For this review, take the finished solid that the model builds, in its own axes (mm). Round coordinates to 2 decimals unless told otherwise and drop trailing zeros. Order: outer loops, then holes, each group sorted by start corner. A loop starts at its lowest first (then second) coordinate and runs counter-clockwise, first axis right, second up. Notation, with made-up numbers: M 41.5,70 L 85.5,70 A21 ccw 85.5,88 Z; hole C 55.25,-23.75 d1. An arc over 180 degrees is marked long. Answer as a JSON object with one key per item and string values.
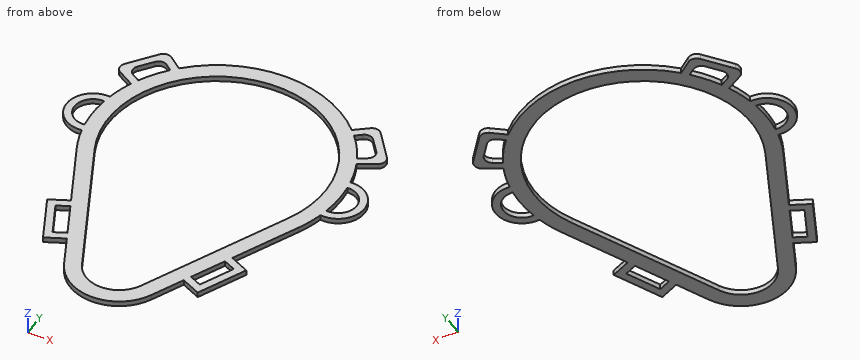
from build123d import *

# Parameters (mm, degrees)
BOSS_EXTRUDE1_DEPTH = 2
BOSS_EXTRUDE2_DEPTH = 2
BOSS_EXTRUDE3_DEPTH = 2
BOSS_EXTRUDE4_DEPTH = 2


with BuildPart() as part:
    # Sketch1 → Boss-Extrude1 (new body)
    with BuildSketch(Plane.XY):
        with BuildLine():
            Line((-42.535849019, -19.992537313), (-16.742834188, -74.869402985))
            ThreePointArc((-16.742834188, -74.869402985), (0, -85.5), (16.742834188, -74.869402985))
            Line((16.742834188, -74.869402985), (42.535849019, -19.992537313))
            ThreePointArc((42.535849019, -19.992537313), (0, 47), (-42.535849019, -19.992537313))
        make_face()
        with BuildLine():
            Line((37.105740634, -17.440298507), (11.312725803, -72.317164179))
            ThreePointArc((11.312725803, -72.317164179), (0, -79.5), (-11.312725803, -72.317164179))
            Line((-11.312725803, -72.317164179), (-37.105740634, -17.440298507))
            ThreePointArc((-37.105740634, -17.440298507), (0, 41), (37.105740634, -17.440298507))
        make_face(mode=Mode.SUBTRACT)
    extrude(amount=BOSS_EXTRUDE1_DEPTH)

    # Sketch2 → Boss-Extrude2 (add)
    # profile 1 of 2: a face of its own
    with BuildSketch(Plane.XY.offset(2)):
        Polygon((38.155605521, -48.118901031), (29.648142834, -66.219262316), (19.692944127, -61.540157838), (28.200406814, -43.439796554), align=None)
        Polygon((29.639341604, -47.430970149), (34.164431925, -49.557835821), (28.209208044, -62.22808872), (23.684117723, -60.101223049), align=None, mode=Mode.SUBTRACT)
    # profile 2 of 2: a face of its own
    with BuildSketch(Plane.XY.offset(2)):
        Polygon((-28.200406814, -43.439796554), (-38.155605521, -48.118901031), (-29.648142834, -66.219262316), (-19.692944127, -61.540157838), align=None)
        Polygon((-29.639341604, -47.430970149), (-23.684117723, -60.101223049), (-28.209208044, -62.22808872), (-34.164431925, -49.557835821), align=None, mode=Mode.SUBTRACT)
    extrude(amount=-BOSS_EXTRUDE2_DEPTH)

    # Sketch3 → Boss-Extrude3 (add)
    # profile 1 of 2: a face of its own
    with BuildSketch(Plane.XY.offset(2)):
        with BuildLine():
            Line((-31.151373165, 31.772817784), (-38.114457897, 37.177116489))
            ThreePointArc((-38.114457897, 37.177116489), (-40.329006137, 37.783626199), (-42.323795344, 36.64657125))
            Line((-42.323795344, 36.64657125), (-50.184128352, 26.519047267))
            ThreePointArc((-50.184128352, 26.519047267), (-50.760622602, 24.115277799), (-49.336666072, 22.094683561))
            Line((-49.336666072, 22.094683561), (-41.03528616, 17.205385487))
            Line((-41.03528616, 17.205385487), (-31.151373165, 31.772817784))
        make_face()
        with BuildLine():
            Line((-35.213971315, 31.128382936), (-37.583912658, 32.967779041))
            ThreePointArc((-37.583912658, 32.967779041), (-39.798460899, 33.574288752), (-41.793250106, 32.437233803))
            Line((-41.793250106, 32.437233803), (-45.72341661, 27.373471811))
            ThreePointArc((-45.72341661, 27.373471811), (-46.29991086, 24.969702343), (-44.87595433, 22.949108105))
            Line((-44.87595433, 22.949108105), (-41.937721652, 21.218565047))
            Line((-41.937721652, 21.218565047), (-35.213971315, 31.128382936))
        make_face(mode=Mode.SUBTRACT)
    # profile 2 of 2: a face of its own
    with BuildSketch(Plane.XY.offset(2)):
        with BuildLine():
            Line((31.151373165, 31.772817784), (41.03528616, 17.205385487))
            Line((41.03528616, 17.205385487), (49.521231884, 22.082259987))
            ThreePointArc((49.521231884, 22.082259987), (50.972840228, 24.118942465), (50.376596508, 26.547879626))
            Line((50.376596508, 26.547879626), (42.329184832, 36.691250185))
            ThreePointArc((42.329184832, 36.691250185), (40.338269585, 37.80509541), (38.139596853, 37.19662773))
            Line((38.139596853, 37.19662773), (31.151373165, 31.772817784))
        make_face()
        with BuildLine():
            Line((35.213971315, 31.128382936), (41.937721652, 21.218565047))
            Line((41.937721652, 21.218565047), (44.9588763, 22.954823155))
            ThreePointArc((44.9588763, 22.954823155), (46.410484644, 24.991505634), (45.814240924, 27.420442794))
            Line((45.814240924, 27.420442794), (41.798639593, 32.481912737))
            ThreePointArc((41.798639593, 32.481912737), (39.807724347, 33.595757962), (37.609051614, 32.987290283))
            Line((37.609051614, 32.987290283), (35.213971315, 31.128382936))
        make_face(mode=Mode.SUBTRACT)
    extrude(amount=-BOSS_EXTRUDE3_DEPTH)

    # Sketch4 → Boss-Extrude4 (add)
    # profile 1 of 2: a face of its own
    with BuildSketch(Plane.XY.offset(2)):
        with BuildLine():
            Line((42.848392472, 8.262286082), (42.848392472, -9.939496711))
            ThreePointArc((42.848392472, -9.939496711), (56.992517927, -0.838605315), (42.848392472, 8.262286082))
        make_face()
        with BuildLine():
            Line((45.848392472, 6.067260087), (45.848392472, -7.744470716))
            ThreePointArc((45.848392472, -7.744470716), (53.992517927, -0.838605315), (45.848392472, 6.067260087))
        make_face(mode=Mode.SUBTRACT)
    # profile 2 of 2: a face of its own
    with BuildSketch(Plane.XY.offset(2)):
        with BuildLine():
            Line((-42.848392472, 8.262286082), (-42.848392472, -9.939496711))
            ThreePointArc((-42.848392472, -9.939496711), (-56.992517927, -0.838605315), (-42.848392472, 8.262286082))
        make_face()
        with BuildLine():
            Line((-45.848392472, 6.067260087), (-45.848392472, -7.744470716))
            ThreePointArc((-45.848392472, -7.744470716), (-53.992517927, -0.838605315), (-45.848392472, 6.067260087))
        make_face(mode=Mode.SUBTRACT)
    extrude(amount=-BOSS_EXTRUDE4_DEPTH)


solid = part.part
1) Add section B-B on y = 0. State the section outline as (x, z) points, and give its area (3 significant figures).
Geometry check:
{"outline": "M -56.96,0 L -53.94,0 L -53.94,2 L -56.96,2 Z; M -47,0 L -41,0 L -41,2 L -47,2 Z; M 41,0 L 47,0 L 47,2 L 41,2 Z; M 53.94,0 L 56.96,0 L 56.96,2 L 53.94,2 Z", "area": "36.1 mm²"}
2) Add section D-D on z = 0.5. State how many separate pieces and enclosed holes the cut face has, and give its area (3 significant figures).
Geometry check:
{"separate pieces": "1", "enclosed holes": "7", "area": "2,540 mm²"}
3) For L1, parallel to X at y = 0, z = 1; L2, parallel to Y at x = -31.5, z = 1.25; L3, parallel to X at y = -48.5, z = 1.4, list the stretches that pass through material, from the lowest coordinate up.
Geometry check:
{"L1": "x = -56.96 to -53.94, -47 to -41, 41 to 47, 53.94 to 56.96", "L2": "y = -62.28 to -55.23, -48.31 to -44.99, -43.47 to -29.37, 26.24 to 34.88", "L3": "x = -37.98 to -31.91, -29.14 to -22.51, 22.51 to 29.14, 31.91 to 37.98"}
4) Add section A-A on x = 0. State the section outline as (y, z) points.
Geometry check:
{"outline": "M -85.5,0 L -79.5,0 L -79.5,2 L -85.5,2 Z; M 41,0 L 47,0 L 47,2 L 41,2 Z"}
5) Add section C-C on y = -39. State the section outline as (x, z) points.
Geometry check:
{"outline": "M -33.6,0 L -26.97,0 L -26.97,2 L -33.6,2 Z; M 26.97,0 L 33.6,0 L 33.6,2 L 26.97,2 Z"}
